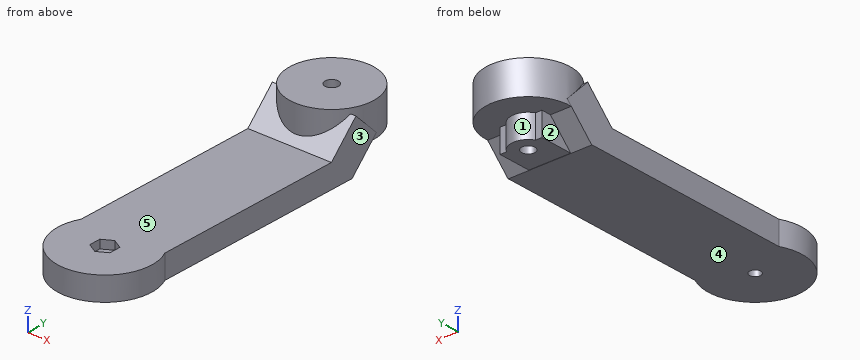
```python
from build123d import *

# Parameters (mm, degrees)
F1_DEPTH  = 7
F2_R      = 12.5
F3_DEPTH  = 10
F4_R      = 2
F5_DEPTH  = 7
F9_W      = 25
F9_H      = 12
F10_DEPTH = 10
F11_R     = 2
F12_DEPTH = 17
F13_R     = 14
F14_DEPTH = 7
F15_R     = 1.65
F16_DEPTH = 7
F18_DEPTH = 2.5


with BuildPart() as f1:
    # F0 (on Top) → F1 (new body)
    with BuildSketch(Plane.XY):
        Polygon((-12.5, -37.5), (12.5, -37.5), (12.5, 37.5), (6.25, 37.5), (-6.25, 37.5), (-12.5, 37.5), align=None)
        with BuildLine():
            Line((-6.25, 37.5), (6.25, 37.5))
            Line((6.25, 37.5), (6.25, 47.5))
            Line((6.25, 47.5), (4.3301270189, 47.5))
            ThreePointArc((4.3301270189, 47.5), (4.8296291314, 46.2940952255), (5, 45))
            ThreePointArc((5, 45), (-1.2940952255, 40.1703708686), (-4.3301270189, 47.5))
            Line((-4.3301270189, 47.5), (-6.25, 47.5))
            Line((-6.25, 47.5), (-6.25, 37.5))
        make_face()
        with BuildLine():
            ThreePointArc((5, 45), (4.8296291314, 46.2940952255), (4.3301270189, 47.5))
            Line((4.3301270189, 47.5), (-4.3301270189, 47.5))
            ThreePointArc((-4.3301270189, 47.5), (-1.2940952255, 40.1703708686), (5, 45))
        make_face()
        with BuildLine():
            Line((-4.3301270189, 47.5), (4.3301270189, 47.5))
            ThreePointArc((4.3301270189, 47.5), (0, 50), (-4.3301270189, 47.5))
        make_face()
    extrude(amount=F1_DEPTH)

    # F2 (on face) → F3 (join)
    with BuildSketch(Plane.XY.offset(7)):
        with Locations((0, 45)):
            Circle(F2_R)
    extrude(amount=F3_DEPTH)

    # F4 (on face) → F5 (cut, through all)
    with BuildSketch(Plane.XY.offset(7)):
        with Locations((0, -33.5)):
            Circle(F4_R)
    extrude(amount=-F5_DEPTH, mode=Mode.SUBTRACT)

    # F9 (on offset) → F10 (join)
    with BuildSketch(Plane(origin=(0, 11.7144660941, -11.7144660941), x_dir=(1, 0, 0), z_dir=(0, -0.7071067812, 0.7071067812))):
        with Locations((0, 32.4662517628)):
            Rectangle(F9_W, F9_H)
    extrude(amount=-F10_DEPTH)

    # F11 (on face) → F12 (cut, through all)
    with BuildSketch(Plane.XY.offset(17)):
        with Locations((0, 45)):
            Circle(F11_R)
    extrude(amount=-F12_DEPTH, mode=Mode.SUBTRACT)

    # F13 (on face) → F14 (join, through all)
    with BuildSketch(Plane(origin=(0, 0, 0), x_dir=(1, 0, 0), z_dir=(0, 0, -1))):
        with Locations((0, 33.5)):
            Circle(F13_R)
    extrude(amount=-F14_DEPTH)

    # F15 (on face) → F16 (cut, through all)
    with BuildSketch(Plane.XY.offset(7)):
        with Locations((0, -33.5)):
            Circle(F15_R)
    extrude(amount=-F16_DEPTH, mode=Mode.SUBTRACT)

    # F17 (on face) → F18 (cut)
    with BuildSketch(Plane.XY.offset(7)):
        Polygon((0, -36.9641016151), (3, -35.2320508076), (3, -31.7679491924), (0, -30.0358983849), (-3, -31.7679491924), (-3, -35.2320508076), align=None)
    extrude(amount=-F18_DEPTH, mode=Mode.SUBTRACT)


solid = f1.part
```
Geometry: final body of the model. Coordinates: model frame, mm. Face numbers are marked on the shaded views. A direction names the side the tool comes from. Coordinates: 2 decimals unless noted, no trailing zeros. Order: outer loops, then holes, each group sorted by start corner. A loop starts at its lowest first (then second) coordinate and runs counter-clockwise, first axis right, second up. Notation, with made-up numbers: (67.25, 55.5) - (89.25, 55.5) arc R20 cw to (89.25, 84.5) - close; hole circle Ø11 at (-1, -13.75). An arc over 180 degrees is marked (long way). Return JSON: item names as keys, results as strings. Group by question number.
1. Material intervals for line 1 along Y through (x, z) = (0, 13.75); line 2 along X through (y, z) = (0.5, 6.5); line 3 along Z through (x, y) = (10, -2), sorted ascending. Write a range as [from, to].
2. Cut plane D-D (z = 13.75). Output: boundary loops of the cut face in (x, y), plus the area to 3 significant figures.
3. Set-up query: the marked faces 1, 2, 3, 4 and 5. Return all of +Z, -Z, +X, -X, +Y, -Y with unobstructed straight access to the full face (end or side cutting, diameter ignored); none if empty.
4. Cut plane B-B (z = 3.25). Output: boundary loops of the cut face in (x, y).
5. Pin query (flat end, axial travel): pin 1 (4 mm diameter, centred on x = -6.5, y = 19, fed in from -Z); pin 2 (8 mm diameter, centred on y = 4.5, z = 8, fed in from +X); pin 3 (3.5 mm diameter, centred on y = 44.5, z = 2.5, fed in from -X). Return the tip coordinate at first contact, or that it passes through.
6. Cut plane C-C (x = 8.75). Output: boundary loops of the cut face in (y, z).
7. Cut plane A-A (y = -33.5). Output: boundary loops of the cut face in (x, z).
Resolved:
{
 "1": {"line 1": "y = [32.5, 43], [47, 57.5]", "line 2": "x = [-12.5, 12.5]", "line 3": "z = [0, 7]"},
 "2": {"outline": "(-12.5, 37.18) - (-9.75, 37.18) arc R12.5 ccw to (9.75, 37.18) - (12.5, 37.18) - (12.5, 40.65) - (11.72, 40.65) arc R12.5 ccw (long way) to (-11.72, 40.65) - (-12.5, 40.65) - close; hole circle Ø4 at (0, 45)", "area": "490 mm²"},
 "3": {"face 1": "-Z, +Y", "face 2": "-Z, -X, +Y", "face 3": "+Z, -Z, +X, +Y", "face 4": "-Z, +X, -X, -Y", "face 5": "+Z, +X, -X, -Y"},
 "4": {"outline": "(-12.5, -27.2) arc R14 ccw (long way) to (12.5, -27.2) - (12.5, 40.82) - (6.25, 40.82) - (6.25, 47.5) - (4.33, 47.5) arc R5 ccw to (-4.33, 47.5) - (-6.25, 47.5) - (-6.25, 40.82) - (-12.5, 40.82) - close; hole circle Ø4 at (0, 45); hole circle Ø3.3 at (0, -33.5)"},
 "5": {"pin 1": "stops at z = 0", "pin 2": "stops at x = 12.5", "pin 3": "stops at x = -6.25"},
 "6": {"outline": "(-44.43, 0) - (37.43, 0) - (37.5, -0.07) - (44.57, 7) - (53.93, 7) - (53.93, 17) - (36.07, 17) - (36.07, 12.64) - (30.43, 7) - (-44.43, 7) - close"},
 "7": {"outline": "(-14, 0) - (-1.65, 0) - (-1.65, 4.5) - (-3, 4.5) - (-3, 7) - (-14, 7) - close; (1.65, 0) - (14, 0) - (14, 7) - (3, 7) - (3, 4.5) - (1.65, 4.5) - close"}
}
